Input: part model. Units: mm. Frame: model coordinates. A direction names the side the tool comes from. Coordinates: 2 decimals unless noted, no trailing zeros. Loops run counter-clockwise (first coordinate to the right, second up) from the corner with the lowest first, then second, coordinate; pieces in that order, holes last. Notation, with made-up numbers: (47, 8) - (82, 8) arc R23 cw to (82, 21) - close; hole circle Ø10 at (30, -24.75). An arc over 180 degrees is marked (long way). Use a Markdown table: item, result. Add a question column.
1. Contact query for a flat-ended pin moving along its axis: P1, Ø1.4, axis at x = -6.5, z = 2.5, coming from the +Y side. Output: stop coordinate, or through.
2. Section query C-C on z = 1. Return the cut outline in (x, y), then the cut area to 3 significant figures.
3. Section query A-A on y = 0. Return the cut outline in (x, z), then the cut area to 3 significant figures.
4. Access query for faces 1 (the face through (-4.45, 4.43, 2.02)), 2 (the face through (-1.3, 4.375, 0.292)), 3 (the face through (1.22, 26.55, 2.02)). Directions: +Z, -Z, +X, -X, +Y, -Y. A direction counts if a zero-diameter tool reaches every point of the face in a straight line with its end or side. Return the directions, or none.
5. Draft query along Y for faces 4 (the face through (3.43, 29.4, 2.02)), 5 (the face through (-1.22, 26.55, 2.02)), 6 (the face through (-3, -4, 2)). Return one class per face: released by +Y, released by -Y, zero draft, split by the parting line, or undercut.
6. Section query B-B on x = -14. Return the cut outline in (y, z), then the cut area to 3 significant figures.
7. Ray query, L1, parallel to X at y = 11, z = 2.25; L2, parallel to Y at x = -14, z = 1.15. Return the intervals inside material, ascending. Write a range as [from, to].
```python
from build123d import *

# Parameters (mm, degrees)
BOX001001004_W     = 3.3
BOX001001004_H     = 23
BOX001001004_DEPTH = 10
FILLET003_R        = 1.5
BOX001001005_W     = 8
BOX001001005_H     = 34
BOX001001005_DEPTH = 4
BOX001001006_W     = 8
BOX001001006_H     = 8
BOX001001006_DEPTH = 4
FILLET_R           = 2
FILLET004_R        = 1.5
CHAMFER005_SIZE    = 0.4
TUBE001_R          = 7
TUBE001_R_2        = 4
TUBE001_DEPTH      = 4
CHAMFER004_SIZE    = 0.4


with BuildPart() as fillet003:
    # Box001001004 → Box001001004 (new body)
    with BuildSketch(Plane(origin=(-1.65, 4, 0), x_dir=(1, 0, 0), z_dir=(0, 0, 1))):
        with Locations((1.65, 11.5)):
            Rectangle(BOX001001004_W, BOX001001004_H)
    extrude(amount=BOX001001004_DEPTH)

    # Fillet003
    fillet003_edges = [fillet003.edges().sort_by_distance(p)[0] for p in [
        (-1.65, 4, 5),
        (-1.65, 27, 5),
        (1.65, 4, 5),
        (1.65, 27, 5),
    ]]
    fillet(fillet003_edges, radius=FILLET003_R)


with BuildPart() as cube007:
    # Box001001005 → Box001001005 (new body)
    with BuildSketch(Plane(origin=(-4, -4, 0), x_dir=(1, 0, 0), z_dir=(0, 0, 1))):
        with Locations((4, 17)):
            Rectangle(BOX001001005_W, BOX001001005_H)
    extrude(amount=BOX001001005_DEPTH)


with BuildPart() as chamfer005:
    # Box001001006 → Box001001006 (new body)
    with BuildSketch(Plane(origin=(-9, -4, 0), x_dir=(1, 0, 0), z_dir=(0, 0, 1))):
        with Locations((4, 4)):
            Rectangle(BOX001001006_W, BOX001001006_H)
    extrude(amount=BOX001001006_DEPTH)

    # Fusion002: union Cube007
    add(cube007.part)

    # Fillet
    fillet_edges = [chamfer005.edges().sort_by_distance(p)[0] for p in [
        (-4, 30, 2),
        (4, -4, 2),
        (4, 30, 2),
    ]]
    fillet(fillet_edges, radius=FILLET_R)

    # Fillet004
    fillet004_edges = [chamfer005.edges().sort_by_distance(p)[0] for p in [
        (-4, 4, 2),
    ]]
    fillet(fillet004_edges, radius=FILLET004_R)

    # Cut002008023012009006003002007005: cut Fillet003
    add(fillet003.part, mode=Mode.SUBTRACT)

    # Chamfer005
    chamfer005_edges = [chamfer005.edges().sort_by_distance(p)[0] for p in [
        (-4, 16.75, 4),
        (-4, 16.75, 0),
        (-4.43934, 4.43934, 4),
        (-4.43934, 4.43934, 0),
        (-3.414214, 29.414214, 0),
        (-3.414214, 29.414214, 4),
        (0, 30, 0),
        (0, 30, 4),
        (3.414214, 29.414214, 0),
        (3.414214, 29.414214, 4),
        (4, 13, 4),
        (4, 13, 0),
        (3.414214, -3.414214, 0),
        (3.414214, -3.414214, 4),
        (-7.25, 4, 0),
        (-7.25, 4, 4),
        (-9, 0, 4),
        (-9, 0, 0),
        (-3.5, -4, 4),
        (-1.21066, 4.43934, 4),
        (-1.65, 15.5, 4),
        (-1.21066, 26.56066, 4),
        (0, 27, 4),
        (1.21066, 26.56066, 4),
        (1.65, 15.5, 4),
        (1.21066, 4.43934, 4),
        (0, 4, 4),
        (-1.21066, 4.43934, 0),
        (0, 4, 0),
        (1.21066, 4.43934, 0),
        (1.65, 15.5, 0),
        (1.21066, 26.56066, 0),
        (0, 27, 0),
        (-1.21066, 26.56066, 0),
        (-1.65, 15.5, 0),
        (-3.5, -4, 0),
    ]]
    chamfer(chamfer005_edges, length=CHAMFER005_SIZE)


with BuildPart() as fusion003001:
    # Tube001 → Tube001 (new body)
    with BuildSketch(Plane.XY):
        Circle(TUBE001_R)
        Circle(TUBE001_R_2, mode=Mode.SUBTRACT)
    extrude(amount=TUBE001_DEPTH)

    # Chamfer004
    chamfer004_edges = [fusion003001.edges().sort_by_distance(p)[0] for p in [
        (-7, 0, 4),
        (-7, 0, 0),
        (-4, 0, 4),
        (-4, 0, 0),
    ]]
    chamfer(chamfer004_edges, length=CHAMFER004_SIZE)


with BuildPart() as fusion003001_1:
    # Chamfer004 placement: moved
    add(fusion003001.part.moved(Location((-14, 0, 0))))

    # Fusion003: union Chamfer005
    add(chamfer005.part)


solid = fusion003001_1.part
```
Resolved:
| question | item | result |
|---|---|---|
| 1 | P1 | y = 4 |
| 2 | outline | (-8.26, -4) - (2, -4) arc R2 ccw to (4, -2) - (4, 28) arc R2 ccw to (2, 30) - (-2, 30) arc R2 ccw to (-4, 28) - (-4, 5.5) arc R1.5 cw to (-5.5, 4) - (-8.26, 4) arc R7 ccw (long way) to start; hole circle Ø8 at (-14, 0); hole (-1.65, 5.5) arc R1.5 ccw to (-0.15, 4) - (0.15, 4) arc R1.5 ccw to (1.65, 5.5) - (1.65, 25.5) arc R1.5 ccw to (0.15, 27) - (-0.15, 27) arc R1.5 ccw to (-1.65, 25.5) - close |
| 2 | area | 327 mm² |
| 3 | outline | (-21, 0.4) - (-20.6, 0) - (-18.4, 0) - (-18, 0.4) - (-18, 3.6) - (-18.4, 4) - (-20.6, 4) - (-21, 3.6) - close; (-10, 0.4) - (-9.6, 0) - (3.6, 0) - (4, 0.4) - (4, 3.6) - (3.6, 4) - (-9.6, 4) - (-10, 3.6) - close |
| 3 | area | 67.4 mm² |
| 4 | face 1 | +Z, -Z, +Y |
| 4 | face 2 | -Z |
| 4 | face 3 | +Z, -Z |
| 5 | face 4 | released by +Y |
| 5 | face 5 | undercut |
| 5 | face 6 | released by -Y |
| 6 | outline | (-7, 0.4) - (-6.6, 0) - (-4.4, 0) - (-4, 0.4) - (-4, 3.6) - (-4.4, 4) - (-6.6, 4) - (-7, 3.6) - close; (4, 0.4) - (4.4, 0) - (6.6, 0) - (7, 0.4) - (7, 3.6) - (6.6, 4) - (4.4, 4) - (4, 3.6) - close |
| 6 | area | 23.4 mm² |
| 7 | L1 | [-4, -1.65], [1.65, 4] |
| 7 | L2 | [-7, -4], [4, 7] |
